Work out the finished part from the listing and answer in its coordinate system (mm). Give positions to 0.01 mm unless a question says otherwise; leave off trailing zeros. Write each loop counter-clockwise with the first axis right and the second up, starting at its lowest first coordinate (ties: lowest second). Pieces come first, ordered by that corner, then holes. Notation, with made-up numbers: (76, -19.75) -> (86, -19.75) arc R17 ccw to (86, -12.75) -> close; hole circle Ø4 at (-24.75, 19). An arc over 180 degrees is marked (long way). Use a Markdown table: item, result. Add a question column.
Q1. Section A-A, the plane z = -12 is taken. Give the vertices of the cut face in (x, y), plus the area to 4 significant figures.
Q2. Section D-D, the plane y = 13.25 is taken. Give the vertices of the cut face in (x, z) (3 decimals).
Q3. Section B-B, the plane x = 70 is taken. Give the vertices of the cut face in (y, z), plus the area to 3 significant figures.
Q4. Section C-C, the plane z = -16.5 is taken. Give the vertices of the cut face in (x, y), plus the area to 3 significant figures.
Q5. Consider line 1 (X direction, y = 7, z = -12); line 2 (X direction, y = 11.25, z = -16.5); line 3 (X direction, y = 9.75, z = -14.75). Determine where each line is inside the solid, lowest interval first.
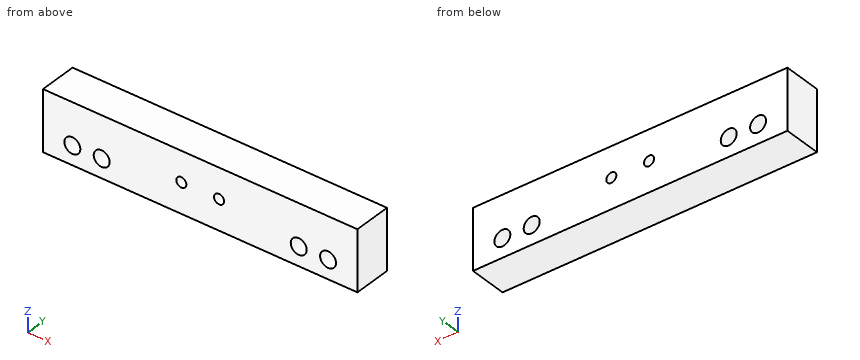
from build123d import *

# Parameters (mm, degrees)
SKETCH1_W           = 125
SKETCH1_H           = 24
BOSS_EXTRUDE1_DEPTH = 15
SKETCH2_R           = 3.175
CUT_EXTRUDE1_DEPTH  = 129.163957492
SKETCH5_R           = 2
CUT_EXTRUDE2_DEPTH  = 129.163957492


with BuildPart() as part:
    # Sketch1 → Boss-Extrude1 (new body)
    with BuildSketch(Plane(origin=(0, 0, 0), x_dir=(1, 0, 0), z_dir=(0, 1, 0))):
        with Locations((62.5, 12)):
            Rectangle(SKETCH1_W, SKETCH1_H)
    extrude(amount=BOSS_EXTRUDE1_DEPTH)

    # Sketch2 → Cut-Extrude1 (cut, symmetric)
    with BuildSketch(Plane(origin=(0, 15, 0), x_dir=(1, 0, 0), z_dir=(0, 1, 0))):
        with Locations(Location((113.333333333, 16.5, 0), (0, 0, 270))):
            Circle(SKETCH2_R)
        with Locations(Location((101.666666667, 16.5, 0), (0, 0, 270))):
            Circle(SKETCH2_R)
    cut_extrude1 = extrude(amount=CUT_EXTRUDE1_DEPTH, both=True, mode=Mode.SUBTRACT)

    # Mirror1: Cut-Extrude1 across plane
    add(cut_extrude1.mirror(Plane.ZY.offset(-62.5)), mode=Mode.SUBTRACT)

    # Sketch5 → Cut-Extrude2 (cut, through all)
    with BuildSketch(Plane(origin=(0, 15, 0), x_dir=(1, 0, 0), z_dir=(0, 1, 0))):
        with Locations(Location((70, 12, 0), (0, 0, 270))):
            Circle(SKETCH5_R)
    cut_extrude2 = extrude(amount=-CUT_EXTRUDE2_DEPTH, mode=Mode.SUBTRACT)

    # Mirror2: Cut-Extrude2 across plane
    add(cut_extrude2.mirror(Plane.ZY.offset(-62.5)), mode=Mode.SUBTRACT)


solid = part.part
Result set:
| question | item | result |
|---|---|---|
| 1 | outline | (0, 0) -> (53, 0) -> (53, 15) -> (0, 15) -> close; (57, 0) -> (68, 0) -> (68, 15) -> (57, 15) -> close; (72, 0) -> (125, 0) -> (125, 15) -> (72, 15) -> close |
| 1 | area | 1,755 mm2 |
| 2 | outline | (0, -24) -> (125, -24) -> (125, 0) -> (0, 0) -> close; hole circle Ø6.35 at (11.667, -16.5); hole circle Ø6.35 at (23.333, -16.5); hole circle Ø4 at (55, -12); hole circle Ø4 at (70, -12); hole circle Ø6.35 at (101.667, -16.5); hole circle Ø6.35 at (113.333, -16.5) |
| 3 | outline | (0, -24) -> (15, -24) -> (15, -14) -> (0, -14) -> close; (0, -10) -> (15, -10) -> (15, 0) -> (0, 0) -> close |
| 3 | area | 300 mm2 |
| 4 | outline | (0, 0) -> (8.49, 0) -> (8.49, 15) -> (0, 15) -> close; (14.84, 0) -> (20.16, 0) -> (20.16, 15) -> (14.84, 15) -> close; (26.51, 0) -> (98.49, 0) -> (98.49, 15) -> (26.51, 15) -> close; (104.84, 0) -> (110.16, 0) -> (110.16, 15) -> (104.84, 15) -> close; (116.51, 0) -> (125, 0) -> (125, 15) -> (116.51, 15) -> close |
| 4 | area | 1,490 mm2 |
| 5 | line 1 | x = 0 to 53, 57 to 68, 72 to 125 |
| 5 | line 2 | x = 0 to 8.49, 14.84 to 20.16, 26.51 to 98.49, 104.84 to 110.16, 116.51 to 125 |
| 5 | line 3 | x = 0 to 9.02, 14.32 to 20.68, 25.98 to 99.02, 104.32 to 110.68, 115.98 to 125 |
